Geometry check sheet. Reference: the model listing, model coordinates, mm. Give positions to 0.01 mm unless a question says otherwise; leave off trailing zeros. Loops run counter-clockwise (first coordinate to the right, second up) from the corner with the lowest first, then second, coordinate; pieces in that order, holes last.
1. Cross-section at A-A, the plane y = 36. Record the cut outline in (x, z).
2. Go/stop test with flat-tipped pins: pin 1 Ø1.5 at (x, y) = (18, 21.5) entering from -Z; pin 2 Ø1.5 at (y, z) = (27.5, 9) entering from +X; pin 3 Ø1 at (x, y) = (-10.5, 16.5) entering from -Z. Record where each tip stops, or that it passes through.
3. Material ranges on L1, parallel to X at y = 2, z = 0 (1 decimal); L2, parallel to X at y = 4, z = 0; L3, parallel to X at y = 4.25, z = 0, recorded low to high.
4. Cross-section at B-B, the plane y = 22.5. Record the cut outline in (x, z).
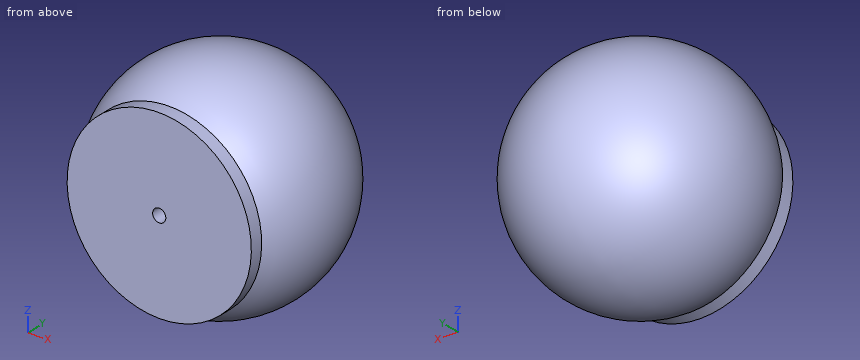
from build123d import *


with BuildPart() as part:
    # Sketch1 → Revolve1 (revolve)
    with BuildSketch(Plane.XY, mode=Mode.PRIVATE) as revolve1_sk:
        with BuildLine():
            Line((-1.5875, 0), (-22.225, 0))
            Line((-22.225, 0), (-22.225, 3.175))
            ThreePointArc((-22.225, 3.175), (-24.066125336, 31.265144421), (0, 45.868827772))
            Line((0, 45.868827772), (0, 42.813696551))
            Line((0, 42.813696551), (-6.35, 42.813696551))
            Line((-6.35, 42.813696551), (-21.1836, 21.629120278))
            Line((-21.1836, 21.629120278), (-25.374009401, 15.644595445))
            Line((-25.374009401, 15.644595445), (-21.1836, 3.175))
            Line((-21.1836, 3.175), (-21.1836, 2.1082))
            Line((-21.1836, 2.1082), (-6.35, 2.1082))
            Line((-6.35, 2.1082), (-6.35, 6.35))
            Line((-6.35, 6.35), (-1.5875, 6.35))
            Line((-1.5875, 6.35), (-1.5875, 2.1082))
            Line((-1.5875, 2.1082), (-1.5875, 0))
        make_face()
    revolve(revolve1_sk.sketch.rotate(Axis((0, 0, 0), (0, 1, 0)), 270), axis=Axis((0, 0, 0), (0, 1, 0)))


solid = part.part
Result:
1. outline: circle Ø41.86 at (0, 0); hole circle Ø22.24 at (0, 0)
2. pin 1: stops at z = -20.77
2. pin 2: stops at x = 24.43
2. pin 3: stops at z = -25.13
3. L1: x = -22.2 to -1.6, 1.6 to 22.2
3. L2: x = -22.78 to -21.46, -6.35 to -1.59, 1.59 to 6.35, 21.46 to 22.78
3. L3: x = -22.94 to -21.54, -6.35 to -1.59, 1.59 to 6.35, 21.54 to 22.94
4. outline: circle Ø53.74 at (0, 0); hole circle Ø41.15 at (0, 0)
